Check sheet for the drawn part. Datum: minimum x, y, z corner. Units: mm. Coordinates: 2 decimals unless noted, no trailing zeros. Loops run counter-clockwise (first coordinate to the right, second up) from the corner with the lowest first, then second, coordinate; pieces in that order, holes last.
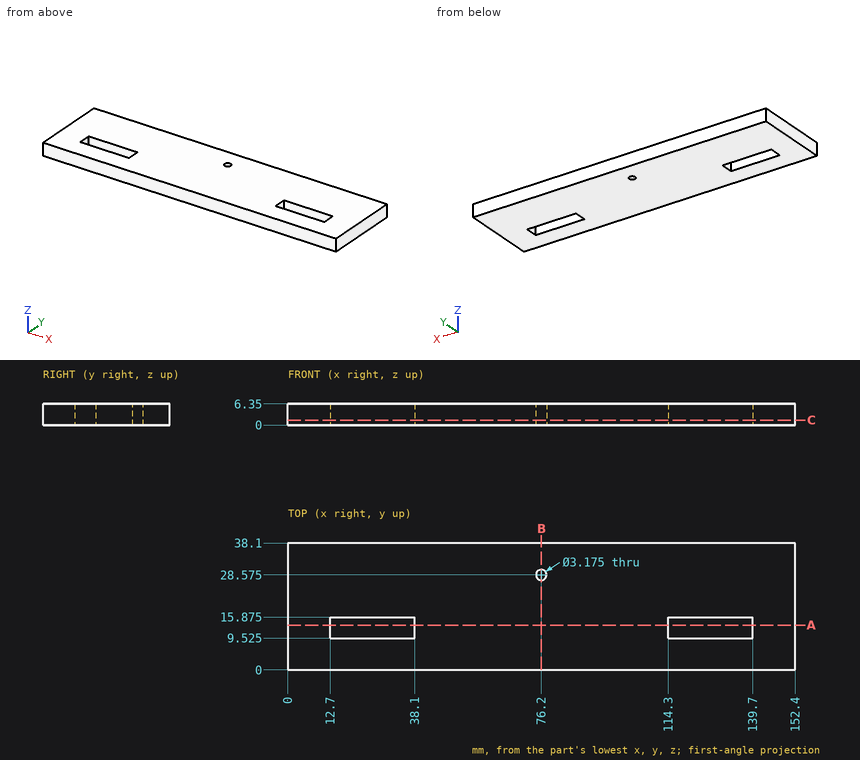
1) Section check B-B on x = 76.2. Enter the section's corners in (y, z).
Answer sheet:
outline: (0, 0) - (26.99, 0) - (26.99, 6.35) - (0, 6.35) - close; (30.16, 0) - (38.1, 0) - (38.1, 6.35) - (30.16, 6.35) - close
2) Section check C-C on z = 1.5. Enter the section's corners in (x, y) (1 decimal).
Answer sheet:
outline: (0, 0) - (152.4, 0) - (152.4, 38.1) - (0, 38.1) - close; hole (12.7, 9.5) - (38.1, 9.5) - (38.1, 15.9) - (12.7, 15.9) - close; hole circle Ø3.2 at (76.2, 28.6); hole (114.3, 9.5) - (139.7, 9.5) - (139.7, 15.9) - (114.3, 15.9) - close
3) Scan lines: line 1 (Y direction, x = 23, z = 5.75) (3 decimals); line 2 (Y direction, x = 76.2, z = 2.25). Record each from-to range of solid material in increasing order.
Answer sheet:
line 1: y = 0 to 9.525, 15.875 to 38.1
line 2: y = 0 to 26.99, 30.16 to 38.1
4) Section check A-A on y = 13.5. Enter the section's corners in (x, z).
Answer sheet:
outline: (0, 0) - (12.7, 0) - (12.7, 6.35) - (0, 6.35) - close; (38.1, 0) - (114.3, 0) - (114.3, 6.35) - (38.1, 6.35) - close; (139.7, 0) - (152.4, 0) - (152.4, 6.35) - (139.7, 6.35) - close
